from build123d import *

# Parameters (mm, degrees)
F0_R     = 20.32
F1_DEPTH = 10.16
F2_R     = 18.415
F3_DEPTH = 12.7
F4_R     = 0.2032


with BuildPart() as f1:
    # F0 (on Top) → F1 (new body)
    with BuildSketch(Plane.XY):
        Circle(F0_R)
    extrude(amount=F1_DEPTH)

    # F2 (on Top) → F3 (cut, symmetric)
    with BuildSketch(Plane.XY):
        Circle(F2_R)
    extrude(amount=F3_DEPTH, both=True, mode=Mode.SUBTRACT)

    # F4
    f4_edges = [f1.edges().sort_by_distance(p)[0] for p in [
        (-20.32, 0, 10.16),
        (-18.415, 0, 10.16),
        (-20.32, 0, 0),
        (-18.415, 0, 0),
    ]]
    fillet(f4_edges, radius=F4_R)


solid = f1.part
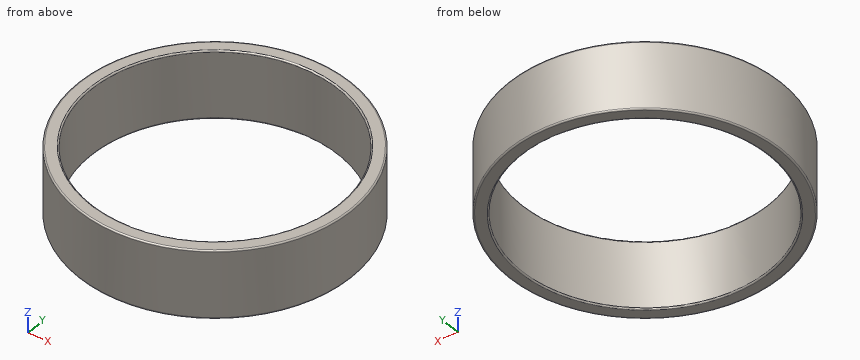
For this review, take the finished solid that the model builds, in its own axes (mm). Round coordinates to 2 decimals unless told otherwise and drop trailing zeros. Loops run counter-clockwise (first coordinate to the right, second up) from the corner with the lowest first, then second, coordinate; pieces in that order, holes last. Notation, with made-up numbers: (-20.5, 75) - (-11.5, 75) arc R5 ccw to (-11.5, 79) - close; hole circle Ø11 at (52.25, 28.5). An arc over 180 degrees is marked (long way). Use one line per item in the form item = value.
Item 1: Consider section C-C on z = 1.75. Write out the cut boundary in (x, y) (3 decimals).
Answers:
outline = circle Ø40.64 at (0, 0); hole circle Ø36.83 at (0, 0)
Item 2: Consider section A-A on x = 0. Write out the cut boundary in (y, z) (3 decimals), then the cut area to 3 significant figures.
Answers:
outline = (-20.32, 0.203) arc R0.203 ccw to (-20.117, 0) - (-18.618, 0) arc R0.203 ccw to (-18.415, 0.203) - (-18.415, 9.957) arc R0.203 ccw to (-18.618, 10.16) - (-20.117, 10.16) arc R0.203 ccw to (-20.32, 9.957) - close; (18.415, 0.203) arc R0.203 ccw to (18.618, 0) - (20.117, 0) arc R0.203 ccw to (20.32, 0.203) - (20.32, 9.957) arc R0.203 ccw to (20.117, 10.16) - (18.618, 10.16) arc R0.203 ccw to (18.415, 9.957) - close
area = 38.6 mm^2
Item 3: Clearance check with flat-ended pins moving along their axes: P1, Ø1.5, axis at y = -13, z = 6, coming from the -X side; P2, Ø3, axis at y = 2.5, z = 8.5, coming from the +X side; P3, Ø1, axis at y = 11.5, z = 9, coming from the +X side. State where each tip first meets the part, or that it passes through.
Answers:
P1 = -16.21
P2 = 20.3
P3 = 17.09
Item 4: For line 1 (Y direction, x = 0, z = 2.5) (3 decimals); line 2 (Y direction, x = -2, z = 1); line 3 (X direction, y = -14.5, z = 3), list the stretches that pass through material, from the lowest coordinate up.
Answers:
line_1 = -20.32 to -18.415, 18.415 to 20.32
line_2 = -20.22 to -18.31, 18.31 to 20.22
line_3 = -14.24 to -11.35, 11.35 to 14.24
